Input: part model. Units: mm. Frame: model coordinates. A direction names the side the tool comes from. Give positions to 0.01 mm unless a question says otherwise; leave off trailing zeros. Write each loop counter-clockwise with the first axis right and the second up, starting at its lowest first coordinate (ties: lowest second). Pieces come first, ordered by that corner, then holes. Notation, with made-up numbers: (66, 79.25) -> (106, 79.25) arc R18 ccw to (106, 109.25) -> close; hole circle Ø1 at (3.5, -38). An arc over 180 degrees is marked (long way). Return JSON: item names as keys, results as strings. Group by question number.
Item 1: Line query: line 1 (Z direction, x = 0, y = 94.25); line 2 (Z direction, x = -3.25, y = 72.5); line 3 (X direction, y = 14.5, z = -0.75). Output: solid intervals per line, ascending. Write a range as [from, to].
Item 2: Set-up query: faces 4 (the face through (0, 25.4, 0)), 5 (the face through (-3, 114.3, 0)), 6 (the face through (0, 88.9, 0)). Return all of +Z, -Z, +X, -X, +Y, -Y with unobstructed straight access to the full face (end or side cutting, diameter ignored); none if empty.
Item 3: Section C-C, the plane y = 103.5. Return loops of the section in (x, z).
Item 4: Pin query (flat end, axial travel): P1, Ø6, axis at y = 52.5, z = 3.5, coming from the -X side; P2, Ø1.5, axis at x = -0.5, z = 0.5, coming from the +Y side; P3, Ø6, axis at x = 4, y = 24.5, coming from the +Z side. Return the tip coordinate at first contact, or that it passes through.
Item 5: Section A-A, the plane x = 0. Return loops of the section in (y, z), then the cut area to 3 significant figures.
Item 6: Section B-B, the plane z = 0. Return loops of the section in (x, y).
Item 7: Mould query, pull axis Z, two halves, no side actions, for faces 1 (the face through (-3, 0, 0)), 2 (the face through (1.38, 56.35, 6.2)), 3 (the face through (2.435, 12.522, 0.767)). Classes: released by +Z, released by -Z, zero draft, split by the parting line, or undercut.
Item 8: Section D-D, the plane y = 48.5. Return loops of the section in (x, z).
Autodesk Inventor part; units mm, degrees
ref_plane "YZ Plane" through (0, 0, 0) normal (1, 0, 0) x (0, 1, 0)
ref_plane "XZ Plane" through (0, 0, 0) normal (0, 1, 0) x (-1, 0, 0)
ref_plane "XY Plane" through (0, 0, 0) normal (0, 0, 1) x (1, 0, 0)
sketch "Sketch1" plane through (0, 0, 0) normal (0, 1, 0) x (-1, 0, 0)
  circle A0 centre (0, 0) radius 6.35
  dimension "d0" = 12.7
extrude "Extrusion1" add sketch "Sketch1" along normal blind 114.3
sketch "Sketch2" plane through (0, 0, 0) normal (0, -1, 0) x (1, 0, 0)
  circle A0 centre (0, 0) radius 2.5527
  dimension "d3" = 5.1054
sketch "Sketch3" plane through (0, 114.3, 0) normal (0, 1, 0) x (1, 0, 0)
  circle A0 centre (0, 0) radius 2.5527
  dimension "d4" = 5.1054
extrude "Extrusion2" cut sketch "Sketch3" against normal blind 25.4
extrude "Extrusion3" cut sketch "Sketch2" against normal blind 25.4
properties part number "INDX_002_Standoff" material "Aluminum 6061"
Answer below:
{
 "1": {"line 1": "z = [-6.35, -2.55], [2.55, 6.35]", "line 2": "z = [-5.46, 5.46]", "line 3": "x = [-6.31, -2.44], [2.44, 6.31]"},
 "2": {"face 4": "-Y", "face 5": "+Z, -Z, +X, -X, +Y", "face 6": "+Y"},
 "3": {"outline": "circle Ø12.7 at (0, 0); hole circle Ø5.11 at (0, 0)"},
 "4": {"P1": "stops at x = -6.33", "P2": "stops at y = 88.9", "P3": "stops at z = 6.27"},
 "5": {"outline": "(0, -6.35) -> (114.3, -6.35) -> (114.3, -2.55) -> (88.9, -2.55) -> (88.9, 2.55) -> (114.3, 2.55) -> (114.3, 6.35) -> (0, 6.35) -> (0, 2.55) -> (25.4, 2.55) -> (25.4, -2.55) -> (0, -2.55) -> close", "area": "1,190 mm2"},
 "6": {"outline": "(-6.35, 0) -> (-2.55, 0) -> (-2.55, 25.4) -> (2.55, 25.4) -> (2.55, 0) -> (6.35, 0) -> (6.35, 114.3) -> (2.55, 114.3) -> (2.55, 88.9) -> (-2.55, 88.9) -> (-2.55, 114.3) -> (-6.35, 114.3) -> close"},
 "7": {"face 1": "zero draft", "face 2": "split by the parting line", "face 3": "undercut"},
 "8": {"outline": "circle Ø12.7 at (0, 0)"}
}
